Input: part model. Units: mm. Frame: model coordinates. Coordinates: 2 decimals unless noted, no trailing zeros. Write each loop counter-clockwise with the first axis right and the second up, starting at its lowest first coordinate (ties: lowest second). Pieces come first, ordered by that corner, then holes. Notation, with made-up numbers: (89.5, 38.5) - (116.5, 38.5) arc R30 cw to (116.5, 61.5) - close; hole circle Ø3 at (85, 76). An arc over 180 degrees is marked (long way). One line per question, with ' | ' between items. Start each with the question number.
1) First-contact query: P1, Ø1.5, axis at x = -18, y = 55.5, coming from the -Z side; P2, Ø6, axis at y = 16, z = 17, coming from the -X side; P3, Ø12, axis at y = 9.5, z = -8.5, coming from the -X side. Flat tips, straight axial feed; report the tip coordinate or a pass-through.
2) Line query: line 1 (X direction, y = 57, z = 0); line 2 (Z direction, x = -1, y = 14.5). Output: solid intervals per line, ascending.
3) Section query A-A on x = 9. Return loops of the section in (y, z) (3 decimals).
4) Section query B-B on z = -9. Return loops of the section in (x, y) (3 decimals), and give its area (3 significant figures).
5) Section query C-C on y = 47. Return loops of the section in (x, z) (1 decimal), and give its area (3 significant figures).
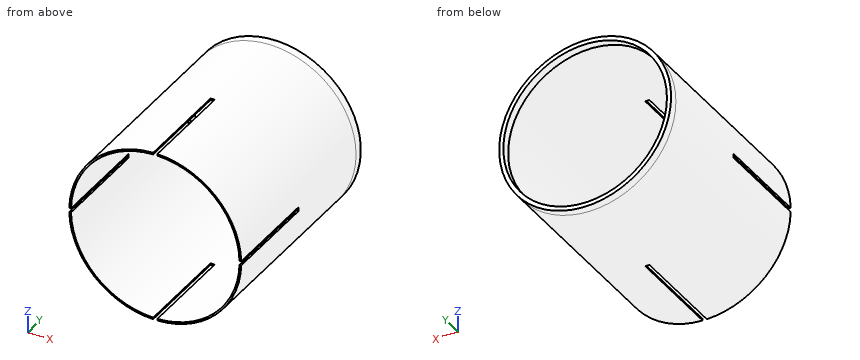
```python
from build123d import *

# Parameters (mm, degrees)
F0_R     = 32.7025
F0_R_2   = 32.0675
F1_DEPTH = 76.2
F3_DEPTH = 38.1
F4_R     = 32.7025
F4_R_2   = 31.115
F5_DEPTH = 3.175


with BuildPart() as f1:
    # F0 (on Front) → F1 (new body)
    with BuildSketch(Plane.XZ):
        Circle(F0_R)
        Circle(F0_R_2, mode=Mode.SUBTRACT)
    extrude(amount=-F1_DEPTH)

    # F2 (on Front) → F3 (cut)
    with BuildSketch(Plane.XZ):
        Polygon((0.79375, 0.79375), (0.79375, 51.373329), (-0.79375, 51.373329), (-0.79375, 0.79375), (-50.8, 0.79375), (-50.8, -0.79375), (-0.79375, -0.79375), (-0.79375, -42.451348), (0.79375, -42.451348), (0.79375, -0.79375), (50.8, -0.79375), (50.8, 0.79375), align=None)
    extrude(amount=-F3_DEPTH, mode=Mode.SUBTRACT)

    # F4 (on face) → F5 (join)
    with BuildSketch(Plane(origin=(0, 76.2, 0), x_dir=(-1, 0, 0), z_dir=(0, 1, 0))):
        Circle(F4_R)
        Circle(F4_R_2, mode=Mode.SUBTRACT)
    extrude(amount=F5_DEPTH)


solid = f1.part
```
Answer key:
1) P1: z = -27.78 | P2: x = -29.55 | P3: x = -32.61
2) line 1: -32.7 to -32.07, 32.07 to 32.7 | line 2: -32.69 to -32.05, 32.05 to 32.69
3) outline: (0, -31.44) - (79.375, -31.44) - (79.375, -29.785) - (76.2, -29.785) - (76.2, -30.779) - (0, -30.779) - close; (0, 30.779) - (76.2, 30.779) - (76.2, 29.785) - (79.375, 29.785) - (79.375, 31.44) - (0, 31.44) - close
4) outline: (-31.44, 0) - (-30.779, 0) - (-30.779, 76.2) - (-29.785, 76.2) - (-29.785, 79.375) - (-31.44, 79.375) - close; (29.785, 76.2) - (30.779, 76.2) - (30.779, 0) - (31.44, 0) - (31.44, 79.375) - (29.785, 79.375) - close | area: 111 mm²
5) outline: circle Ø65.4 at (0, 0); hole circle Ø64.1 at (0, 0) | area: 129 mm²
